```python
from build123d import *

# Parameters (mm, degrees)
F3_R      = 4
F4_DEPTH  = 10
F7_DEPTH  = 25
F9_DEPTH  = 25
F10_R     = 1.475
F11_DEPTH = 15
F12_DEPTH = 25


with BuildPart() as f1:
    # F0 (on Front) → F1 (revolve)
    with BuildSketch(Plane.XZ):
        with BuildLine():
            Line((0, 0), (0, 20))
            ThreePointArc((0, 20), (-20, 0), (0, -20))
            Line((0, -20), (0, 0))
        make_face()
    revolve(axis=Axis((0, 0, -10), (0, 0, -1)))

    # F3 (on offset) → F4 (cut)
    with BuildSketch(Plane.XZ.offset(10)):
        with Locations((-8.868288, 5.899725)):
            Circle(F3_R)
        with Locations((8.794304, 6.119836)):
            Circle(F3_R)
    extrude(amount=F4_DEPTH, mode=Mode.SUBTRACT)

    # F6 (on offset) → F7 (cut)
    with BuildSketch(Plane.XZ.offset(17)):
        with BuildLine():
            add(Edge.make_bspline(
                [(-3, 2.491697), (-5.107968, 2.491697), (-4.053984, -1.245848), (-3, -4.983393), (-1.946016, -1.245848), (-0.892032, 2.491697), (-3, 2.491697)],
                knots=[0, 0, 0, 2.094395, 2.094395, 4.18879, 4.18879, 6.283185, 6.283185, 6.283185], degree=2, weights=[1, 0.5, 1, 0.5, 1, 0.5, 1]))
        make_face()
        with BuildLine():
            add(Edge.make_bspline(
                [(3, 2.491697), (0.892032, 2.491697), (1.946016, -1.245848), (3, -4.983393), (4.053984, -1.245848), (5.107968, 2.491697), (3, 2.491697)],
                knots=[0, 0, 0, 2.094395, 2.094395, 4.18879, 4.18879, 6.283185, 6.283185, 6.283185], degree=2, weights=[1, 0.5, 1, 0.5, 1, 0.5, 1]))
        make_face()
    extrude(amount=F7_DEPTH, mode=Mode.SUBTRACT)

    # F8 (on offset) → F9 (cut)
    with BuildSketch(Plane.XZ.offset(10)):
        with BuildLine():
            Line((-12, -9.5), (-12.253571, -9.5))
            ThreePointArc((-12.253571, -9.5), (0, -16), (12.253571, -9.5))
            Line((12.253571, -9.5), (12, -9.5))
            Line((12, -9.5), (9.89303, -6))
            Line((9.89303, -6), (8, -9.5))
            Line((8, -9.5), (6, -6))
            Line((6, -6), (4, -9.5))
            Line((4, -9.5), (2, -6))
            Line((2, -6), (0, -9.5))
            Line((0, -9.5), (-2, -6))
            Line((-2, -6), (-4, -9.5))
            Line((-4, -9.5), (-6, -6))
            Line((-6, -6), (-8, -9.5))
            Line((-8, -9.5), (-10, -6))
            Line((-10, -6), (-12, -9.5))
        make_face()
    extrude(amount=F9_DEPTH, mode=Mode.SUBTRACT)

    # F10 (on Front) → F11 (cut)
    with BuildSketch(Plane.XZ):
        with Locations((-8.868279, 5.899623)):
            Circle(F10_R)
        with Locations((8.771721, 5.899623)):
            Circle(F10_R)
    extrude(amount=-F11_DEPTH, mode=Mode.SUBTRACT)

    # F10 (on Front) → F12 (cut)
    with BuildSketch(Plane.XZ):
        with Locations((-8.868279, 5.899623)):
            Circle(F10_R)
        with Locations((8.771721, 5.899623)):
            Circle(F10_R)
    extrude(amount=F12_DEPTH, mode=Mode.SUBTRACT)


solid = f1.part
```
Geometry check sheet. Reference: the model listing, model coordinates, mm. Coordinates: 2 decimals unless noted, no trailing zeros. Loops run counter-clockwise (first coordinate to the right, second up) from the corner with the lowest first, then second, coordinate; pieces in that order, holes last.
Item 1: Sectioned sample at C-C, the plane x = -16. Record the boundary of the cut face in (y, z).
Item 2: Thickness scan on line 1 (X direction, y = -11, z = 7.5); line 2 (X direction, y = 7, z = 6); line 3 (Z direction, x = 7.5, y = -10.5) (3 decimals). Record the ranges inside material, lowest first.
Item 3: Sectioned sample at B-B, the plane z = 12. Record the boundary of the cut face in (x, y).
Item 4: Sectioned sample at D-D, the plane y = 11.5. Record the boundary of the cut face in (x, z) (3 decimals), then the cut area to 3 significant figures.
Item 5: Sectioned sample at A-A, the plane y = -12. Record the boundary of the cut face in (x, z).
Item 6: Go/stop test with flat-tipped pins: pin 1 Ø8 at (x, z) = (-4.5, 7.5) entering from -Y; pin 2 Ø0.7 at (x, z) = (-3.5, 1) entering from -Y; pin 3 Ø4 at (y, z) = (7.5, -3) entering from +X. Record where each tip stops, or that it passes through.
Check result:
1. outline: circle Ø24 at (0, 0)
2. line 1: x = -14.92 to -12.53, -5.2 to 5.04, 12.55 to 14.92
2. line 2: x = -17.75 to -10.34, -7.4 to 7.3, 10.24 to 17.75
2. line 3: z = -15.281 to -13.959, -8.625 to 2.335, 9.905 to 15.281
3. outline: circle Ø32 at (0, 0)
4. outline: circle Ø32.726 at (0, 0); hole circle Ø2.95 at (-8.868, 5.9); hole circle Ø2.95 at (8.772, 5.9)
4. area: 827 mm2
5. outline: circle Ø32 at (0, 0); hole circle Ø8 at (-8.87, 5.9); hole (-12.25, -9.5) arc R14.8 ccw to (12.25, -9.5) - (12, -9.5) - (9.89, -6) - (8, -9.5) - (6, -6) - (4, -9.5) - (2, -6) - (0, -9.5) - (-2, -6) - (-4, -9.5) - (-6, -6) - (-8, -9.5) - (-10, -6) - (-12, -9.5) - close; hole circle Ø8 at (8.79, 6.12)
6. pin 1: stops at y = -19.43
6. pin 2: stops at y = -17
6. pin 3: stops at x = 19.05
